Autodesk Inventor part; units mm, degrees
ref_plane "YZ Plane" through (0, 0, 0) normal (1, 0, 0) x (0, 1, 0)
ref_plane "XZ Plane" through (0, 0, 0) normal (0, 1, 0) x (-1, 0, 0)
ref_plane "XY Plane" through (0, 0, 0) normal (0, 0, 1) x (1, 0, 0)
sketch "Sketch1" plane through (0, 0, 0) normal (0, 0, 1) x (1, 0, 0)
  line L0 (-22.8574, 44.4294) -> (22.8574, 44.4294)
  line L1 (10.3429, -56) -> (10.3429, -59)
  line L2 (2.65, -59) -> (2.65, -56)
  line L3 (2.65, -56) -> (1.5, -56)
  line L4 (1.5, -56) -> (1.5, -54)
  line L5 (1.5, -54) -> (2.65, -54)
  line L6 (2.65, -54) -> (2.65, -51.6)
  line L7 (2.65, -51.6) -> (1.5, -51.6)
  line L8 (1.5, -51.6) -> (1.5, -51)
  line L9 (1.5, -51) -> (-1.5, -51)
  line L10 (-1.5, -51) -> (-1.5, -51.6)
  line L11 (-1.5, -51.6) -> (-2.65, -51.6)
  line L12 (-2.65, -51.6) -> (-2.65, -54)
  line L13 (-2.65, -54) -> (-1.5, -54)
  line L14 (-1.5, -56) -> (-2.65, -56)
  line L15 (-1.5, -54) -> (-1.5, -56)
  line L16 (-2.65, -56) -> (-2.65, -59)
  line L17 (-10.3429, -56) -> (-10.3429, -59)
  line L18 (0, -51.179) -> (0, -65.7621) construction
  line L19 (10.3429, -59) -> (2.65, -59)
  line L20 (-2.65, -59) -> (-10.3429, -59)
  line L21 (-24.2882, 0) -> (26.7754, 0) construction
  circle A0 centre (0, -24.4294) radius 3.9
  circle A1 centre (0, 24.4294) radius 3.9
  line L22 (22.8574, -56) -> (22.8574, -34.4294)
  line L23 (22.8574, -34.4294) -> (25.8574, -34.4294)
  line L24 (25.8574, -27.0794) -> (22.8574, -27.0794)
  line L25 (22.8574, -27.0794) -> (22.8574, -25.9294)
  line L26 (22.8574, -25.9294) -> (20.8574, -25.9294)
  line L27 (20.8574, -25.9294) -> (20.8574, -27.0794)
  line L28 (20.8574, -27.0794) -> (18.4574, -27.0794)
  line L29 (18.4574, -27.0794) -> (18.4574, -25.9294)
  line L30 (18.4574, -25.9294) -> (17.8574, -25.9294)
  line L31 (17.8574, -25.9294) -> (17.8574, -22.9294)
  line L32 (17.8574, -22.9294) -> (18.4574, -22.9294)
  line L33 (18.4574, -22.9294) -> (18.4574, -21.7794)
  line L34 (18.4574, -21.7794) -> (20.8574, -21.7794)
  line L35 (20.8574, -21.7794) -> (20.8574, -22.9294)
  line L36 (20.8574, -22.9294) -> (22.8574, -22.9294)
  line L37 (22.8574, -22.9294) -> (22.8574, -21.7794)
  line L38 (22.8574, -21.7794) -> (25.8574, -21.7794)
  line L39 (22.8574, -56) -> (10.3429, -56)
  line L40 (39.0531, -24.4294) -> (-31.8887, -24.4294) construction
  line L41 (25.8574, -14.4294) -> (22.8574, -14.4294)
  line L42 (25.8574, -27.0794) -> (25.8574, -34.4294)
  line L43 (25.8574, -14.4294) -> (25.8574, -21.7794)
  line L44 (22.8574, 44.4294) -> (22.8574, 34.4294)
  line L45 (22.8574, 34.4294) -> (25.8574, 34.4294)
  line L46 (25.8574, 27.0794) -> (22.8574, 27.0794)
  line L47 (22.8574, 27.0794) -> (22.8574, 25.9294)
  line L48 (22.8574, 25.9294) -> (20.8574, 25.9294)
  line L49 (20.8574, 25.9294) -> (20.8574, 27.0794)
  line L50 (20.8574, 27.0794) -> (18.4574, 27.0794)
  line L51 (18.4574, 27.0794) -> (18.4574, 25.9294)
  line L52 (18.4574, 25.9294) -> (17.8574, 25.9294)
  line L53 (17.8574, 25.9294) -> (17.8574, 22.9294)
  line L54 (17.8574, 22.9294) -> (18.4574, 22.9294)
  line L55 (18.4574, 22.9294) -> (18.4574, 21.7794)
  line L56 (18.4574, 21.7794) -> (20.8574, 21.7794)
  line L57 (20.8574, 21.7794) -> (20.8574, 22.9294)
  line L58 (20.8574, 22.9294) -> (22.8574, 22.9294)
  line L59 (22.8574, 22.9294) -> (22.8574, 21.7794)
  line L60 (22.8574, 21.7794) -> (25.8574, 21.7794)
  line L61 (25.8574, 14.4294) -> (22.8574, 14.4294)
  line L62 (25.8574, 27.0794) -> (25.8574, 34.4294)
  line L63 (25.8574, 14.4294) -> (25.8574, 21.7794)
  line L64 (22.8574, 14.4294) -> (22.8574, -14.4294)
  line L65 (0, 77.8205) -> (0, -95.1737) construction
  line L66 (-22.8574, -56) -> (-22.8574, -34.4294)
  line L67 (-22.8574, -34.4294) -> (-25.8574, -34.4294)
  line L68 (-25.8574, -27.0794) -> (-22.8574, -27.0794)
  line L69 (-22.8574, -27.0794) -> (-22.8574, -25.9294)
  line L70 (-22.8574, -25.9294) -> (-20.8574, -25.9294)
  line L71 (-20.8574, -25.9294) -> (-20.8574, -27.0794)
  line L72 (-20.8574, -27.0794) -> (-18.4574, -27.0794)
  line L73 (-18.4574, -27.0794) -> (-18.4574, -25.9294)
  line L74 (-18.4574, -25.9294) -> (-17.8574, -25.9294)
  line L75 (-17.8574, -25.9294) -> (-17.8574, -22.9294)
  line L76 (-17.8574, -22.9294) -> (-18.4574, -22.9294)
  line L77 (-18.4574, -22.9294) -> (-18.4574, -21.7794)
  line L78 (-18.4574, -21.7794) -> (-20.8574, -21.7794)
  line L79 (-20.8574, -21.7794) -> (-20.8574, -22.9294)
  line L80 (-20.8574, -22.9294) -> (-22.8574, -22.9294)
  line L81 (-22.8574, -22.9294) -> (-22.8574, -21.7794)
  line L82 (-22.8574, -21.7794) -> (-25.8574, -21.7794)
  line L83 (-25.8574, -14.4294) -> (-22.8574, -14.4294)
  line L84 (-25.8574, -27.0794) -> (-25.8574, -34.4294)
  line L85 (-25.8574, -14.4294) -> (-25.8574, -21.7794)
  line L86 (-25.8574, 14.4294) -> (-22.8574, 14.4294)
  line L87 (-25.8574, 14.4294) -> (-25.8574, 21.7794)
  line L88 (-22.8574, 21.7794) -> (-25.8574, 21.7794)
  line L89 (-22.8574, 22.9294) -> (-22.8574, 21.7794)
  line L90 (-20.8574, 22.9294) -> (-22.8574, 22.9294)
  line L91 (-20.8574, 21.7794) -> (-20.8574, 22.9294)
  line L92 (-18.4574, 21.7794) -> (-20.8574, 21.7794)
  line L93 (-18.4574, 22.9294) -> (-18.4574, 21.7794)
  line L94 (-17.8574, 22.9294) -> (-18.4574, 22.9294)
  line L95 (-17.8574, 25.9294) -> (-17.8574, 22.9294)
  line L96 (-18.4574, 25.9294) -> (-17.8574, 25.9294)
  line L97 (-18.4574, 27.0794) -> (-18.4574, 25.9294)
  line L98 (-20.8574, 27.0794) -> (-18.4574, 27.0794)
  line L99 (-20.8574, 25.9294) -> (-20.8574, 27.0794)
  line L100 (-22.8574, 25.9294) -> (-20.8574, 25.9294)
  line L101 (-22.8574, 27.0794) -> (-22.8574, 25.9294)
  line L102 (-25.8574, 27.0794) -> (-22.8574, 27.0794)
  line L103 (-25.8574, 27.0794) -> (-25.8574, 34.4294)
  line L104 (-22.8574, 34.4294) -> (-25.8574, 34.4294)
  line L105 (-22.8574, 44.4294) -> (-22.8574, 34.4294)
  line L106 (-22.8574, 14.4294) -> (-22.8574, -14.4294)
  line L107 (-22.8574, -56) -> (-10.3429, -56)
  line L108 (-37.0496, 24.4294) -> (41.724, 24.4294) construction
  point P0 (0, 0)
  dimension "d4" = 3
  dimension "d6" = 3
  dimension "d7" = 2.4
  dimension "d10" = 5.3
  dimension "d11" = 8
  dimension "d12" = 5
  dimension "d13" = 20.6859
  dimension "d14" = 7.8
  dimension "d15" = 34.5706
  dimension "d16" = 7.8
  dimension "d24" = 3
  dimension "d26" = 51.7147
  dimension "d29" = 48.8588
  dimension "d31" = 3
  dimension "d32" = 8
  dimension "d33" = 5.3
  dimension "d36" = 20
  dimension "d37" = 20
  dimension "d38" = 10
  dimension "d39" = 103.4294
extrude "Extrusion1" add sketch "Sketch1" along normal blind 3
equation "\"d13\" = 0.4 * d26"
properties part number "Y-Shafts-Holder_Front-Outer"
Can you work these out from the model? Positions are in its coordinate system, mm. A direction names the side the tool comes from. Round coordinates to 2 decimals unless told otherwise and drop trailing zeros. Loops run counter-clockwise (first coordinate to the right, second up) from the corner with the lowest first, then second, coordinate; pieces in that order, holes last. Notation, with made-up numbers: (87.5, 11) -> (137.5, 11) arc R32 ccw to (137.5, 50) -> close; hole circle Ø5 at (-5, 16.25). An arc over 180 degrees is marked (long way). One line per item, written item: value. Start each with the question number.
1. If I drill on probe 1 along Y at (x, z) = (-18, 1.85); probe 2 along Y at (x, z) = (0, 0.9); probe 3 along X at (y, z) = (-53, 0.95), over which ranges is the centre line in solid material (lowest first)?
2. If we mould it in two halves opening along Y, with no side actions, what happens to faces 4 (the flat face through (1.5, -55, 1)), 5 (the flat face through (-17.857, -24, 1))? For each: pulls with the +Y half, pulls with the -Y half, needs draft (parallel to the pull), parting line crosses it, or undercut.
3. For pin 1 (0.9 mm diameter, centred on y = 26.5, z = 1, fed in from -X); pin 2 (0.5 mm diameter, centred on x = -18, z = 2, fed in from -Y); pin 3 (1.2 mm diameter, centred on y = -53, z = 2, fed in from +X), each with a flat end and sliding along its axis, tell me the tip position at first contact or that it passes through.
4. If we section it at A-A, the plane x = 0: Write out the boundary of the cut face in (y, z).
5. If we section it at C-C, the plane z = 0.9: Give the number of separate pieces and of enclosed holes in the cut face, then the cut area to 3 significant figures.
6. For faces 1 (the flat face through (22.857, 39, 1)), 2 (the flat face through (-22, -22.929, 1)), 3 (the flat face through (22, 22.929, 1)), which set-ups out of +Z, -Z, +X, -X, +Y, -Y let a thin tool reach every point of the face, with its end or its side?
7. If we section it at B-B, the plane y = -40: Write out the boundary of the cut face in (x, z).
8. If we section it at D-D, the plane x = 14.5: Write out the boundary of the cut face in (y, z).
Calculated:
1. probe 1: y = -56 to -25.93, -22.93 to 22.93, 25.93 to 44.43
1. probe 2: y = -51 to -28.33, -20.53 to 20.53, 28.33 to 44.43
1. probe 3: x = -22.86 to -2.65, 2.65 to 22.86
2. face 4: needs draft
2. face 5: undercut
3. pin 1: stops at x = -22.86
3. pin 2: stops at y = -56
3. pin 3: stops at x = 22.86
4. outline: (-51, 0) -> (-28.33, 0) -> (-28.33, 3) -> (-51, 3) -> close; (-20.53, 0) -> (20.53, 0) -> (20.53, 3) -> (-20.53, 3) -> close; (28.33, 0) -> (44.43, 0) -> (44.43, 3) -> (28.33, 3) -> close
5. separate pieces: 1
5. enclosed holes: 2
5. area: 4,620 mm²
6. face 1: +Z, -Z, +X, +Y
6. face 2: +Z, -Z, -X
6. face 3: +Z, -Z, +X
7. outline: (-22.86, 0) -> (22.86, 0) -> (22.86, 3) -> (-22.86, 3) -> close
8. outline: (-56, 0) -> (44.43, 0) -> (44.43, 3) -> (-56, 3) -> close
